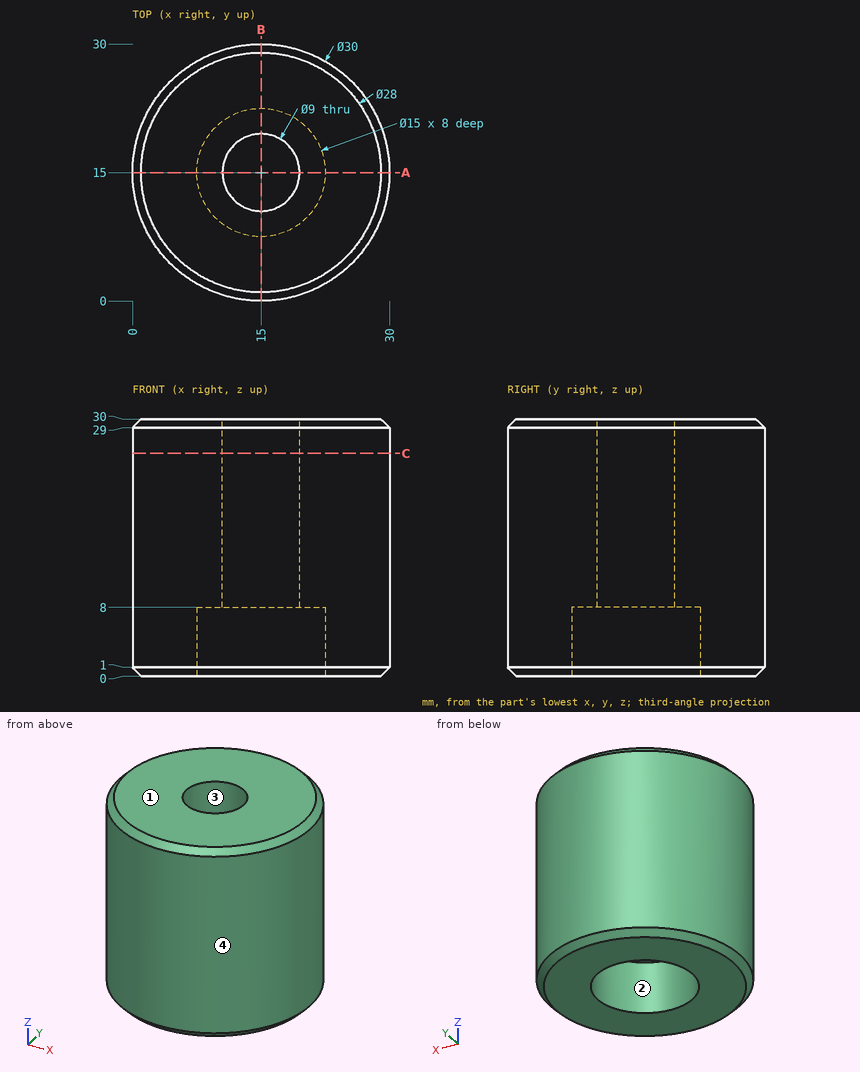
Verification items for this drawing (mm, ordinates from the low corner). Coordinates: 2 decimals unless noted, no trailing zeros. Order: outer loops, then holes, each group sorted by start corner. A loop starts at its lowest first (then second) coordinate and runs counter-clockwise, first axis right, second up. Notation, with made-up numbers: (60.25, 23) - (81.25, 23) arc R11 cw to (81.25, 33) - close; hole circle Ø3 at (13.25, -24). An arc over 180 degrees is marked (long way). Answer as a JSON object with one key per item and string values. Group by question number.
Item 1: Draft check along X on the marked faces 1, 2, 3 and 4. Enter one of: +X half, -X half, draft (parallel to the pull), parting line (faces both ways), or undercut.
Item 2: Sectioned sample at A-A, the plane y = 15. Record the cut outline in (x, z).
Item 3: Depth check by flat-ended pin: pin 1 Ø1 at (y, z) = (21, 3) entering from -X; pin 2 Ø8 at (x, z) = (14.5, 6) entering from +Y; pin 3 Ø10 at (x, z) = (24.5, 3.5) entering from -Y; pin 4 Ø12 at (y, z) = (5.5, 9) entering from +X. Enter the tip coordinate at first touch or a pass-through.
Item 4: Scan lines: probe 1 along Y at (x, z) = (15, 22); probe 2 along Y at (x, z) = (11.25, 11.75); probe 3 along X at (y, z) = (12.5, 2). Record each from-to range of solid material in increasing order.
Item 5: Sectioned sample at C-C, the plane z = 26. Record the cut outline in (x, y).
Resolved:
{
 "1": {"face 1": "draft", "face 2": "undercut", "face 3": "undercut", "face 4": "parting line"},
 "2": {"outline": "(0, 1) - (1, 0) - (7.5, 0) - (7.5, 8) - (10.5, 8) - (10.5, 30) - (1, 30) - (0, 29) - close; (19.5, 8) - (22.5, 8) - (22.5, 0) - (29, 0) - (30, 1) - (30, 29) - (29, 30) - (19.5, 30) - close"},
 "3": {"pin 1": "x = 1.04", "pin 2": "y = 30", "pin 3": "y = 0.69", "pin 4": "x = 29.59"},
 "4": {"probe 1": "0 to 10.5, 19.5 to 30", "probe 2": "0.48 to 12.51, 17.49 to 29.52", "probe 3": "0.21 to 7.93, 22.07 to 29.79"},
 "5": {"outline": "circle Ø30 at (15, 15); hole circle Ø9 at (15, 15)"}
}
